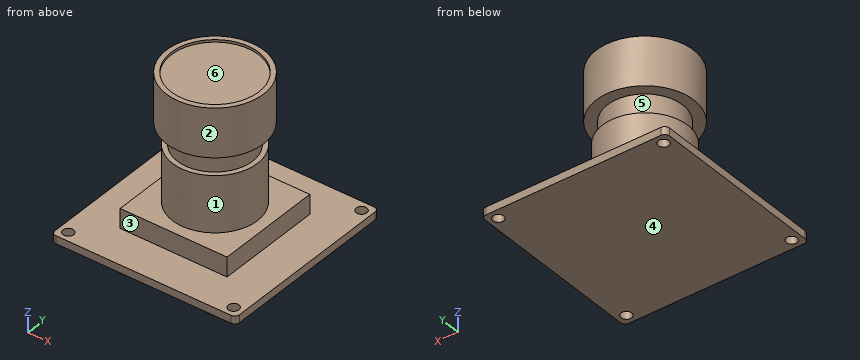
from build123d import *

# Parameters (mm, degrees)
SKETCH_1_W          = 38
SKETCH_1_H          = 38
EXTRUDE_1_DEPTH     = 1.6
SKETCH_2_R          = 1.1
CUT_EXTRUDE_1_DEPTH = 27.917652201
FILLET_1_R          = 1
SKETCH_3_W          = 22
SKETCH_3_H          = 22
EXTRUDE_2_DEPTH     = 4
SKETCH_4_R          = 8.725
EXTRUDE_3_DEPTH     = 15.5
SKETCH_5_R          = 7.725
EXTRUDE_4_DEPTH     = 30
SKETCH_6_R          = 10
EXTRUDE_5_DEPTH     = 10
SKETCH_7_R          = 9
CUT_EXTRUDE_3_DEPTH = 0.5


with BuildPart() as part:
    # 스케치1 → 보스-돌출1 (new body)
    with BuildSketch(Plane.XY):
        Rectangle(SKETCH_1_W, SKETCH_1_H)
    extrude(amount=EXTRUDE_1_DEPTH)

    # 스케치2 → 컷-돌출1 (cut, through all)
    with BuildSketch(Plane.XY.offset(1.6)):
        with Locations((-17, 17)):
            Circle(SKETCH_2_R)
        with Locations((17, -17)):
            Circle(SKETCH_2_R)
        with Locations((17, 17)):
            Circle(SKETCH_2_R)
        with Locations((-17, -17)):
            Circle(SKETCH_2_R)
    extrude(amount=-CUT_EXTRUDE_1_DEPTH, mode=Mode.SUBTRACT)

    # 필렛1
    fillet_1_edges = [part.edges().sort_by_distance(p)[0] for p in [
        (-19, 19, 0.8),
        (19, 19, 0.8),
        (19, -19, 0.8),
        (-19, -19, 0.8),
    ]]
    fillet(fillet_1_edges, radius=FILLET_1_R)

    # 스케치3 → 보스-돌출2 (add)
    with BuildSketch(Plane.XY.offset(1.6)):
        Rectangle(SKETCH_3_W, SKETCH_3_H)
    extrude(amount=EXTRUDE_2_DEPTH)

    # 스케치4 → 보스-돌출3 (add)
    with BuildSketch(Plane.XY.offset(1.6)):
        Circle(SKETCH_4_R)
    extrude(amount=EXTRUDE_3_DEPTH)

    # 스케치5 → 보스-돌출4 (add)
    with BuildSketch(Plane.XY.offset(1.6)):
        Circle(SKETCH_5_R)
    extrude(amount=EXTRUDE_4_DEPTH)

    # 스케치6 → 보스-돌출5 (add)
    with BuildSketch(Plane.XY.offset(31.6)):
        Circle(SKETCH_6_R)
    extrude(amount=-EXTRUDE_5_DEPTH)

    # 스케치7 → 컷-돌출3 (cut)
    with BuildSketch(Plane.XY.offset(31.6)):
        Circle(SKETCH_7_R)
    extrude(amount=-CUT_EXTRUDE_3_DEPTH, mode=Mode.SUBTRACT)


solid = part.part
Verification items for the finished model (mm, model axes). Face numbers are marked on the shaded views. A direction names the side the tool comes from. Give positions to 0.01 mm unless a question says otherwise; leave off trailing zeros. Write each loop counter-clockwise with the first axis right and the second up, starting at its lowest first coordinate (ties: lowest second). Pieces come first, ordered by that corner, then holes. Notation, with made-up numbers: M -8.5,-12 L 21.5,-12 A14 ccw 21.5,13 Z; hole C 49.5,-35.5 d7. An arc over 180 degrees is marked long. Use CSV: the item, a comma, the result in double quotes.
1) Access from +Z, -Z, +X, -X, +Y, -Y to the whole of each face (thin tool, end or side, straight path). Record for the marked faces 1, 2 and 3.
Final values:
face 1,"none"
face 2,"+Z"
face 3,"+Z, +X, -X, -Y"
2) Cross-section at A-A (y = -17). Enter the section's corners in (x, z), plus the area to 3 significant figures.
Final values:
outline,"M -19,0 L -18.1,0 L -18.1,1.6 L -19,1.6 Z; M -15.9,0 L 15.9,0 L 15.9,1.6 L -15.9,1.6 Z; M 18.1,0 L 19,0 L 19,1.6 L 18.1,1.6 Z"
area,"53.8 mm²"
3) Cross-section at D-D (x = 0). Enter the section's corners in (y, z) (3 decimals).
Final values:
outline,"M -19,0 L 19,0 L 19,1.6 L 11,1.6 L 11,5.6 L 8.725,5.6 L 8.725,17.1 L 7.725,17.1 L 7.725,21.6 L 10,21.6 L 10,31.6 L 9,31.6 L 9,31.1 L -9,31.1 L -9,31.6 L -10,31.6 L -10,21.6 L -7.725,21.6 L -7.725,17.1 L -8.725,17.1 L -8.725,5.6 L -11,5.6 L -11,1.6 L -19,1.6 Z"
4) Cross-section at C-C (y = -10.5). Enter the section's corners in (x, z), plus the area to 3 significant figures.
Final values:
outline,"M -19,0 L 19,0 L 19,1.6 L 11,1.6 L 11,5.6 L -11,5.6 L -11,1.6 L -19,1.6 Z"
area,"149 mm²"
5) Material ranges on line 1 along Y through (x, z) = (17, 0.7); line 2 along Z through (x, y) = (1, -9); line 3 along Z through (x, y) = (-6, 15), recorded low to high.
Final values:
line 1,"-19 to -18.1, -15.9 to 15.9, 18.1 to 19"
line 2,"0 to 5.6, 21.6 to 31.6"
line 3,"0 to 1.6"
6) Release check for a two-part mould opening along Y. For the marked faces 4, 5 and 6 record: released by +Y, released by -Y, zero draft, split by the parting line, or undercut.
Final values:
face 4,"zero draft"
face 5,"split by the parting line"
face 6,"undercut"
7) Go/stop test with flat-tipped pins: pin 1 Ø2 at (y, z) = (-11.5, 5.5) entering from +X; pin 2 Ø2 at (y, z) = (-8, 19.5) entering from +X; pin 3 Ø8 at (x, y) = (-13, 10.5) entering from +Z. Record where each tip stops, or that it passes through.
Final values:
pin 1,"x = 11"
pin 2,"x = 3.27"
pin 3,"z = 5.6"
